Autodesk Inventor part; units mm, degrees
ref_plane "Work Plane1" through (17, 0, 0) normal (1, 0, 0) x (0, 0, -1)
ref_plane "YZ Plane" through (0, 0, 0) normal (1, 0, 0) x (0, 1, 0)
ref_plane "XZ Plane" through (0, 0, 0) normal (0, 1, 0) x (-1, 0, 0)
sketch "Sketch1" plane through (0, 0, 0) normal (1, 0, 0) x (0, 1, 0)
  circle A0 centre (0, 0) radius 2.925
  dimension "diameter" = 5.85
extrude "Shaft" add sketch "Sketch1" along normal mid plane 30
sketch "Sketch2" plane through (0, 0, 0) normal (0, 0, 1) x (1, 0, 0)
  line L0 (-15, -2.925) -> (-15, 2.925) construction
  line L1 (15, -2.925) -> (-15, -2.925) construction
  line L2 (15, 2.925) -> (15, -2.925) construction
  line L3 (-15, 2.925) -> (15, 2.925) construction
  line L4 (-15, -2.925) -> (15, -2.925)
  line L5 (-8, -2.925) -> (-8, -2.925)
  line L6 (-15, -2.925) -> (15, -2.925)
  line L7 (-13, 0) -> (-9, 0) construction
  line L8 (-12.1, -0.9) -> (-9.9, -0.9)
  line L9 (-9.9, 0.9) -> (-12.1, 0.9)
  arc A0 (-12.1, 0.9) -> (-12.1, -0.9) centre (-12.1, 0) ccw
  arc A1 (-9.9, -0.9) -> (-9.9, 0.9) centre (-9.9, 0) ccw
  point P0 (0, 0)
  point P1 (15, 0)
  point P2 (-11, 0)
  dimension "d17" = 1.8
  dimension "d20" = 2
  dimension "d21" = 1
  dimension "d22" = 7
extrude "Slot for Differential Gear" cut sketch "Sketch2" along normal through all both and the other way through all
ref_plane "Work Plane1" through (17, 0, 0) normal (1, 0, 0) x (0, 0, -1)
sketch "Sketch3" plane through (17, 0, 0) normal (1, 0, 0) x (0, 0, -1)
  arc A0 (1.6583, -2.5) -> (-1.6583, -2.5) centre (0, 0) ccw construction
  circle A1 centre (0, 0) radius 2.925 construction
  line L0 (-1.6583, -2.5) -> (1.6583, -2.5)
  arc A2 (1.6125, -2.35) -> (-1.6125, -2.35) centre (0, 0) ccw
  line L1 (1.6125, -2.35) -> (-1.6125, -2.35)
  point P0 (-1.5184, -2.5)
  point P1 (1.5184, -2.5)
  dimension "d49" = 3
  dimension "d50" = 2.5
  dimension "wheel_offset" = 0.15
extrude "Wheel Insert Profile" add sketch "Sketch3" along normal blind 12
loft "Loft1" add section 1 edges at (15, -2.925, 0) section 2 edges at (17, -2.35, 0) (17, 2.85, 0)
ref_plane "Work Plane2" through (15, 2.3671, 1.5873) normal (1, 0, 0) x (0, 0, -1)
sketch "Sketch4" plane through (15, 2.3671, 1.5873) normal (1, 0, 0) x (0, 0, -1)
  circle A0 centre (1.5873, -2.3671) radius 3.75
  dimension "d35" = 7.5
extrude "Stopper" add sketch "Sketch4" against normal blind 1
fillet "Fillet1" radius 0.5 2 edges at (15, 0, 3.75) (14, 0, 3.75)
sketch "Sketch8" plane through (-15, 0, 0) normal (-1, 0, 0) x (0, 0, 1)
  circle A0 centre (0, 0) radius 2.925
  circle A1 centre (0, 0) radius 2.7 construction
  circle A2 centre (0, 0) radius 2.65
  dimension "d68" = 5.4
  dimension "d69" = 0.05
extrude "Differential Gear Insert Profile" cut sketch "Sketch8" against normal blind 8
fillet "Fillet3" radius 1 1 edges at (-7, -2.925, 0)
chamfer "Chamfer4" distance 0.5 angle 45 2 edges at (-15, 0, -2.65) (29, 2.85, 0)
properties part number "rear shaft v2"
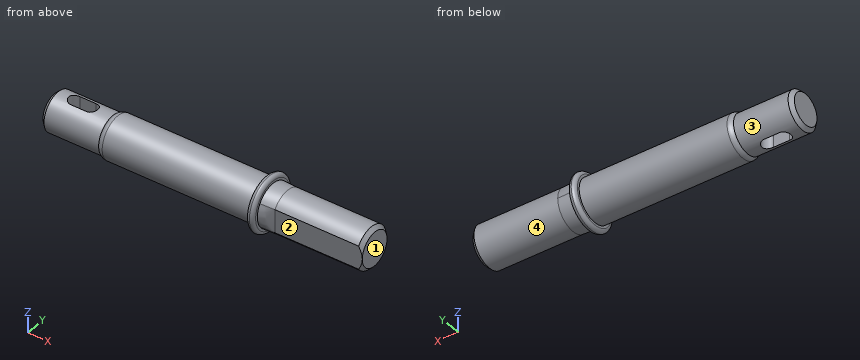
Work out the finished part from the listing and answer in its coordinate system (mm). Face numbers are marked on the shaded views. A direction names the side the tool comes from. Coordinates: 2 decimals unless noted, no trailing zeros. Write each loop counter-clockwise with the first axis right and the second up, starting at its lowest first coordinate (ties: lowest second). Pieces come first, ordered by that corner, then holes. Notation, with made-up numbers: (18, -20.5) - (60, -20.5) arc R16 cw to (60, -14.5) - close; hole circle Ø5 at (45.25, 69). An arc over 180 degrees is marked (long way). Answer as a JSON object with one key per item and string values.
Q1. Given pin 1 Ø2.5 at (x, z) = (-10.5, 0) entering from +Y; pin 2 Ø1.5 at (x, y) = (23, 0.5) entering from +Z; pin 3 Ø2.5 at (x, z) = (25, -0.5) entering from -Y, each flat-ended and moving along its own axis, determine where each tip first touches the part or whether it passes through.
Results list:
{"pin 1": "stops at y = 2.65", "pin 2": "stops at z = 2.85", "pin 3": "stops at y = -2.35"}
Q2. Find section A-A (x = -8.5). Write down the section's boundary in (y, z).
Results list:
{"outline": "circle Ø5.3 at (0, 0)"}
Q3. Consider L1, parallel to Z at x = 10, y = 1.75; L2, parallel to X at y = -0.75, z = 0.25; L3, parallel to X at y = 0.25, z = -3. Determine where each line is inside the solid, lowest interval first. Write a range as from..to.
Results list:
{"L1": "z = -2.34..2.34", "L2": "x = -15..-12.6, -9.4..29", "L3": "x = 14..15"}
Q4. Which of the six approach directions +Z, -Z, +X, -X, +Y, -Y give full straight-line access (tool end or side, diameter ignored) to the marked faces 1, 2, 3 and 4?
Results list:
{"face 1": "+Z, -Z, +X, +Y, -Y", "face 2": "+Z, -Z, +X, -Y", "face 3": "-X", "face 4": "+X"}
Q5. Find section C-C (x = 6). Write down the section's boundary in (y, z) (3 decimals), plus the area to 3 significant figures.
Results list:
{"outline": "circle Ø5.85 at (0, 0)", "area": "26.9 mm^2"}
Q6. Find section B-B (x = 24.5). Write down the section's boundary in (y, z).
Results list:
{"outline": "(-2.35, -1.61) arc R2.85 ccw (long way) to (-2.35, 1.61) - close"}
